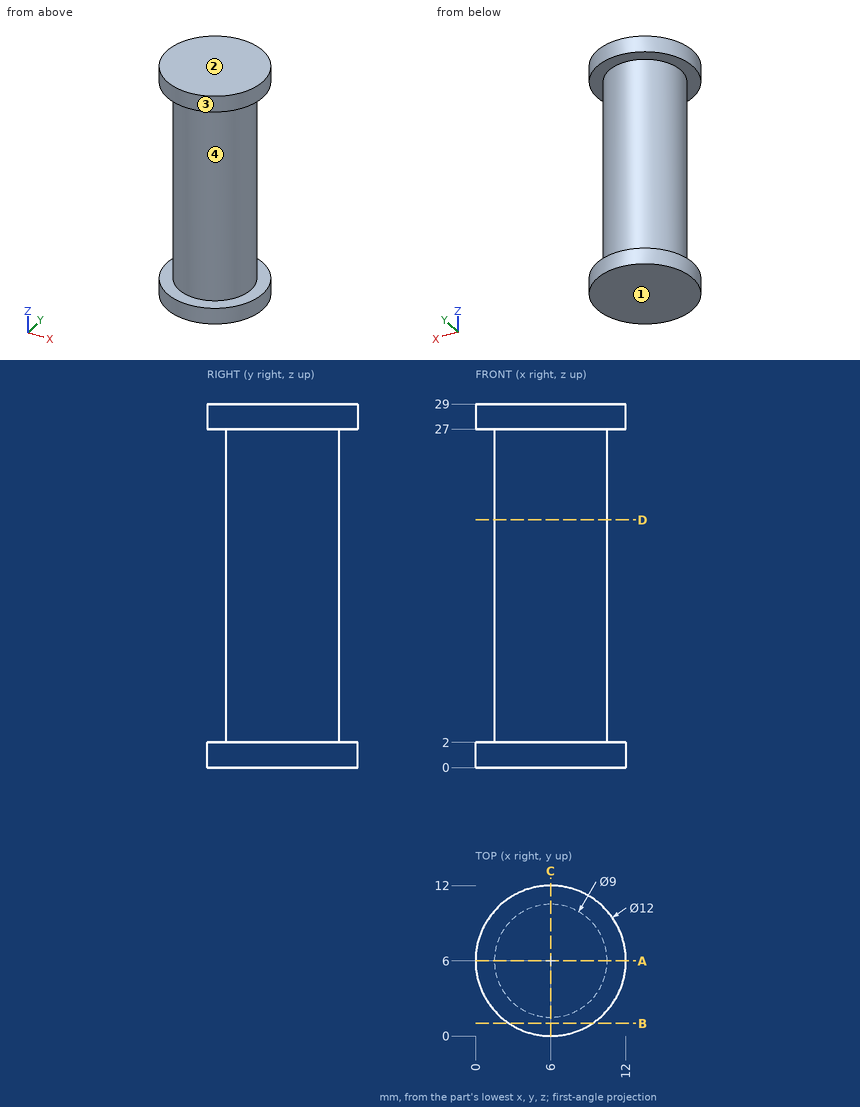
The figure shows three views and two pictorial views of one solid part (mm, origin at its lowest corner). Answer the questions. Give positions to 0.01 mm unless a question says otherwise; leave off trailing zeros. Order: outer loops, then holes, each group sorted by start corner. A loop starts at its lowest first (then second) coordinate and runs counter-clockwise, first axis right, second up. Notation, with made-up numbers: (6.25, -33) -> (14.25, -33) arc R19 ccw to (14.25, -23) -> close; hole circle Ø4 at (35.25, -34.75). An arc over 180 degrees is marked (long way). Answer as CSV lines item,"result". Start each with the question number.
Q1. A cutting plane is placed at D-D (z = 19.75). Determine the outline of the cut face in (x, y).
Q2. Given pin 1 (1 mm diameter, centred on y = 2, z = 25.5, fed in from +X); pin 2 (5 mm diameter, centred on x = 3.5, z = 6.5, fed in from -Y), each flat-ended and moving along its own axis, determine where each tip first touches the part or whether it passes through.
Q3. Find the intervals of material crossed by L1, parallel to Z at x = 6.5, y = 1; L2, parallel to X at y = 2.25, z = 19; L3, parallel to Y at x = 3.5, z = 23.5, in increasing order.
Q4. A cutting plane is placed at B-B (y = 1). Determine the outline of the cut face in (x, z).
Q5. Determine the mould class of the marked faces 1, 2, 3 and 4 for opening direction Z: pulls with the +Z half, pulls with the -Z half, needs draft (parallel to the pull), parting line crosses it, or undercut.
Q6. A cutting plane is placed at A-A (y = 6). Determine the outline of the cut face in (x, z).
Results found:
1,outline,"circle Ø9 at (6, 6)"
2,pin 1,"x = 8.83"
2,pin 2,"y = 1.5"
3,L1,"0 to 2, 27 to 29"
3,L2,"3.51 to 8.49"
3,L3,"2.26 to 9.74"
4,outline,"(2.68, 0) -> (9.32, 0) -> (9.32, 2) -> (2.68, 2) -> close; (2.68, 27) -> (9.32, 27) -> (9.32, 29) -> (2.68, 29) -> close"
5,face 1,"pulls with the -Z half"
5,face 2,"pulls with the +Z half"
5,face 3,"needs draft"
5,face 4,"undercut"
6,outline,"(0, 0) -> (12, 0) -> (12, 2) -> (10.5, 2) -> (10.5, 27) -> (12, 27) -> (12, 29) -> (0, 29) -> (0, 27) -> (1.5, 27) -> (1.5, 2) -> (0, 2) -> close"
